Design review of the part built by this model. Coordinates are the model's own, in mm. A direction names the side the tool comes from. Give positions to 0.01 mm unless a question says otherwise; leave off trailing zeros. Order: outer loops, then holes, each group sorted by start corner. A loop starts at its lowest first (then second) coordinate and runs counter-clockwise, first axis right, second up. Notation, with made-up numbers: M 33,-34 L 50,-34 A11 cw 50,-22 Z; hole C -37.75,-2 d3. An arc over 180 degrees is marked long. Answer as a JSON object with one key per item and string values.
from build123d import *

# Parameters (mm, degrees)
CYLINDER012_R          = 0.6
CYLINDER012_DEPTH      = 20
CYLINDER011_R          = 0.6
CYLINDER011_DEPTH      = 20
BOX010_W               = 20
BOX010_H               = 5
BOX010_DEPTH           = 11
PAD001_DEPTH           = 3
SKETCH005_R            = 4
PAD002_DEPTH           = 8
SKETCH006_R            = 4
PAD003_DEPTH           = 14
BOX009_W               = 20
BOX009_H               = 5
BOX009_DEPTH           = 11
BOX009_PLACEMENT_ANGLE = 14


with BuildPart() as cylinder047:
    # Cylinder012 → Cylinder012 (new body)
    with BuildSketch(Plane(origin=(55, 19, -5), x_dir=(1, 0, 0), z_dir=(0, 0, 1))):
        Circle(CYLINDER012_R)
    extrude(amount=CYLINDER012_DEPTH)


with BuildPart() as cylinder046:
    # Cylinder011 → Cylinder011 (new body)
    with BuildSketch(Plane(origin=(55, -9.5, -5), x_dir=(1, 0, 0), z_dir=(0, 0, 1))):
        Circle(CYLINDER011_R)
    extrude(amount=CYLINDER011_DEPTH)


with BuildPart() as cube010:
    # Box010 → Box010 (new body)
    with BuildSketch(Plane(origin=(45, -12, -0.5), x_dir=(1, 0, 0), z_dir=(0, 0, 1))):
        with Locations((10, 2.5)):
            Rectangle(BOX010_W, BOX010_H)
    extrude(amount=BOX010_DEPTH)


with BuildPart() as pad003:
    # Sketch004 → Pad001 (new body)
    with BuildSketch(Plane.XY.offset(10.5)):
        with BuildLine():
            ThreePointArc((14.120466, 10.991566), (6.522754, -2.168145), (18.163211, -11.935589))
            Line((18.163211, -11.935589), (98.163211, -11.935589))
            ThreePointArc((98.163211, -11.935589), (120.099455, 12.003546), (94.339546, 31.769884))
            Line((14.120466, 10.991566), (94.339546, 31.769884))
        make_face()
    extrude(amount=PAD001_DEPTH)

    # Sketch005 → Pad002 (new body)
    with BuildSketch(Plane(origin=(0, 0, 10.5), x_dir=(1, 0, 0), z_dir=(0, 0, -1))):
        with Locations((98.0594, -10.0638)):
            Circle(SKETCH005_R)
    extrude(amount=PAD002_DEPTH)

    # Sketch006 → Pad003 (new body)
    with BuildSketch(Plane(origin=(0, 0, 10.5), x_dir=(1, 0, 0), z_dir=(0, 0, -1))):
        with Locations((18.0594, 0)):
            Circle(SKETCH006_R)
    extrude(amount=PAD003_DEPTH)


with BuildPart() as tapa_con_taladros:
    # Box009 → Box009 (new body)
    with BuildSketch(Plane.XY):
        with Locations((10, 2.5)):
            Rectangle(BOX009_W, BOX009_H)
    extrude(amount=BOX009_DEPTH)


with BuildPart() as tapa_con_taladros_1:
    # Box009 placement: moved
    add(tapa_con_taladros.part.moved(Location((45, 14, -0.5))).rotate(Axis((45, 14, -0.5), (0, 0, 1)), BOX009_PLACEMENT_ANGLE))

    # Fusion005: union Cube010, Pad003
    add(cube010.part)
    add(pad003.part)

    # Cut011: cut Cylinder046
    add(cylinder046.part, mode=Mode.SUBTRACT)

    # Cut012: cut Cylinder047
    add(cylinder047.part, mode=Mode.SUBTRACT)


with BuildPart() as tapa_con_taladros_2:
    # Cut012 placement: moved
    add(tapa_con_taladros_1.part.moved(Location((-21, -19, 89))))


solid = tapa_con_taladros_2.part
(1) To check wall thickness, follow L1, parallel to X at y = -28.5, z = 98.75; L2, parallel to Y at x = 34, z = 96; L3, parallel to Z at x = 83, y = -17.5. State the ranges of each line that lie inside material, in increasing order. Write a range as from..to.
Checked values:
{"L1": "x = 24..33.4, 34.6..44", "L2": "y = -31..-29.1, -27.9..-26, -2.51..-0.6, 0.6..2.65", "L3": "z = 99.5..102.5"}
(2) We need section D-D (x = 9.5). Write out the cut boundary in (y, z), plus the area to 3 significant figures.
Checked values:
{"outline": "M -30.94,99.5 L -3.77,99.5 L -3.77,102.5 L -30.94,102.5 Z", "area": "81.5 mm^2"}
(3) We need section A-A (z = 97.5). Write out the cut boundary in (x, y).
Checked values:
{"outline": "C -2.94,-19 d8; M 22.79,-0.15 L 24,-5 L 43.41,-0.16 L 42.2,4.69 Z; M 24,-31 L 44,-31 L 44,-26 L 24,-26 Z; C 77.06,-8.94 d8; hole C 34,-28.5 d1.2; hole C 34,0 d1.2"}
(4) We need section B-B (y = -2). Write out the cut boundary in (x, z).
Checked values:
{"outline": "M 16.32,99.5 L 23.25,99.5 L 23.25,88.5 L 36.03,88.5 L 36.03,99.5 L 98.07,99.5 L 98.07,102.5 L 16.32,102.5 Z"}
(5) Draft analysis for pull direction Y (two halves, no side actions). For faces 5 (the flat face through (24, -29, 94)), 6 (the cylindrical face through (-14.515, -20.94, 100.979)), 7 (the flat face through (33.567, -2.615, 93.923)), state which applies: +Y half, -Y half, draft (parallel to the pull), parting line (faces both ways), or undercut.
Checked values:
{"face 5": "draft", "face 6": "parting line", "face 7": "undercut"}
(6) We need section C-C (x = 75.5). Write out the cut boundary in (y, z), plus the area to 3 significant figures.
Checked values:
{"outline": "M -30.94,99.5 L -12.62,99.5 L -12.62,91.5 L -5.25,91.5 L -5.25,99.5 L 13.04,99.5 L 13.04,102.5 L -30.94,102.5 Z", "area": "191 mm^2"}
(7) Tool access review of faces 1 (the flat face through (34, -26, 94)), 2 (the cylindrical face through (80.754, -7.404, 95.556)), 3 (the flat face through (32.668, 2.235, 100.979)), 4 (the flat face through (23.4, -2.6, 93.9)): name each direction out of +Z, -Z, +X, -X, +Y, -Y from which nothing blocks a thin tool from reaching the whole face with its end or side.
Checked values:
{"face 1": "-Z, +X, -X", "face 2": "-Z", "face 3": "+Z, -X, +Y", "face 4": "-Z, -X, -Y"}
(8) Insertion check: pin 1 (2.5 mm diameter, centred on x = 78, y = -10, fed in from -Z); pin 2 (4 mm diameter, centred on x = 48, y = -0.5, fed in from -Z); pin 3 (6 mm diameter, centred on x = 82.5, z = 99.5, fed in from +Y). Each pin has a flat end and moves straight along its axis. Give the tip position at first contact, or say it passes through.
Checked values:
{"pin 1": "stops at z = 91.5", "pin 2": "stops at z = 99.5", "pin 3": "stops at y = 12.98"}
